The drawing under review shows one solid part. Ordinate dimensions are in mm from its lowest x, y, z. A direction names the side the tool comes from. Coordinates: 2 decimals unless noted, no trailing zeros. Order: outer loops, then holes, each group sorted by start corner. A loop starts at its lowest first (then second) coordinate and runs counter-clockwise, first axis right, second up.
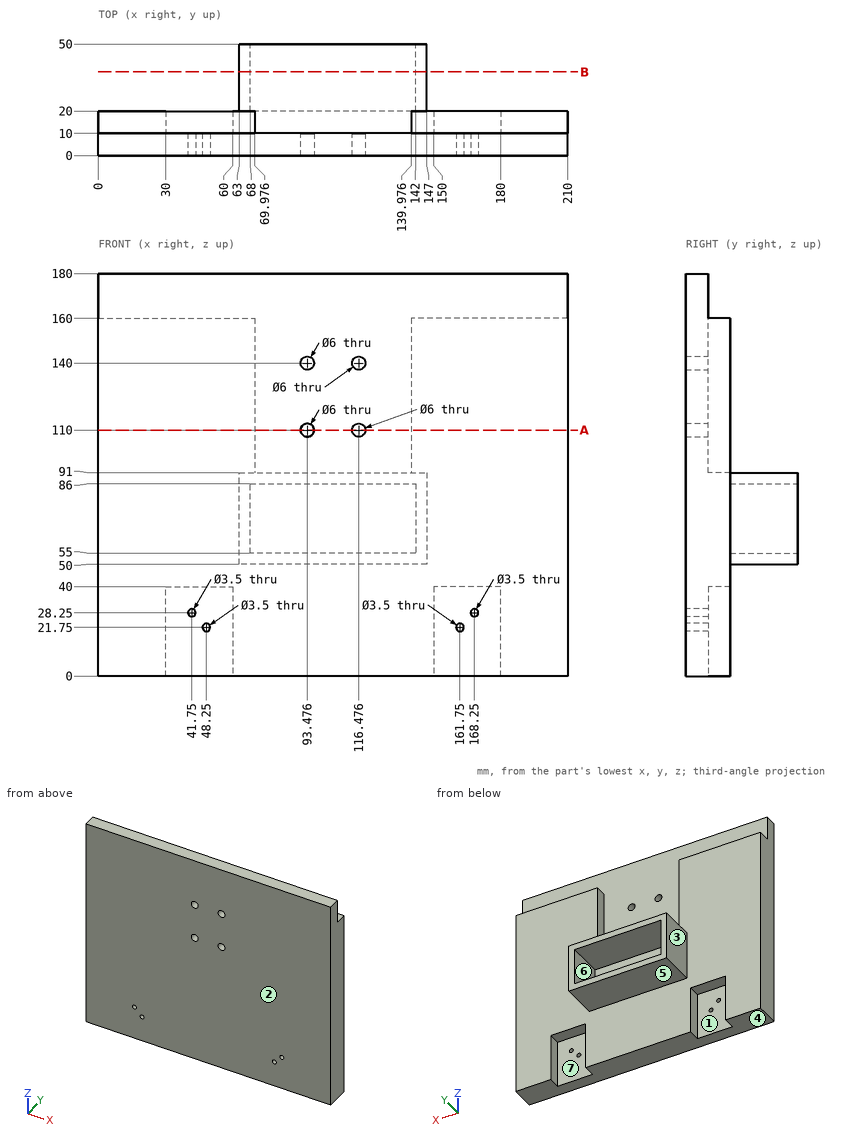
1. The part is to be moulded in two halves that separate along X. For the marked faces 1, 2 and 3, say which applies: +X half, -X half, draft (parallel to the pull), parting line (faces both ways), or undercut.
Answer below:
face 1: undercut
face 2: draft
face 3: -X half
2. Machinability: for the marked faces 4, 5, 6 and 7, which of the approach directions +Z, -Z, +X, -X, +Y, -Y give a long, thin tool a straight path to every point of the face, cutting with its end or side? Answer none if there is none.
Answer below:
face 4: -Z, +X, -X, +Y, -Y
face 5: -Z, +X, -X, +Y
face 6: +Y
face 7: -Z, +Y
3. Take a section at A-A, the plane z = 110. Give the boundary of the cut face in (x, y), plus the area to 3 significant figures.
Answer below:
outline: (0, 0) - (90.48, 0) - (90.48, 10) - (69.98, 10) - (69.98, 20) - (0, 20) - close; (96.48, 0) - (113.48, 0) - (113.48, 10) - (96.48, 10) - close; (119.48, 0) - (210, 0) - (210, 20) - (139.98, 20) - (139.98, 10) - (119.48, 10) - close
area: 3,380 mm2
4. To check wall thickness, follow L1, parallel to X at y = 4.5, z = 21.75; L2, parallel to X at y = 15.5, z = 132; L3, parallel to X at y = 3, z = 110. State the ranges of each line that lie inside material, in increasing order.
Answer below:
L1: x = 0 to 46.5, 50 to 160, 163.5 to 210
L2: x = 0 to 69.98, 139.98 to 210
L3: x = 0 to 90.48, 96.48 to 113.48, 119.48 to 210
5. Take a section at B-B, the plane y = 37.5. Give the boundary of the cut face in (x, z), plus the area to 3 significant figures.
Answer below:
outline: (63, 50) - (147, 50) - (147, 91) - (63, 91) - close; hole (68, 55) - (142, 55) - (142, 86) - (68, 86) - close
area: 1,150 mm2
6. Clearance check with flat-ended pins moving along their axes: pin 1 Ø20 at (x, y) = (124.5, 22) entering from +Z; pin 2 Ø8 at (x, y) = (138, 23) entering from +Z; pin 3 Ø7 at (x, z) = (93.48, 140) entering from +Y. State where each tip first meets the part, or that it passes through.
Answer below:
pin 1: stops at z = 91
pin 2: stops at z = 160
pin 3: stops at y = 10
